```python
from build123d import *

# Parameters (mm, degrees)
CROQUIS1_W              = 20
CROQUIS1_H              = 60
SALIENTE_EXTRUIR1_DEPTH = 31
CORTAR_EXTRUIR1_REACH   = 72.434
CROQUIS2_W              = 21
CROQUIS2_H              = 50
CORTAR_EXTRUIR2_REACH   = 72.434
CROQUIS3_W              = 5
CROQUIS3_H              = 2
CORTAR_EXTRUIR3_REACH   = 72.434
CROQUIS4_W              = 7
CROQUIS4_H              = 2


with BuildPart() as part:
    # Croquis1 → Saliente-Extruir1 (new body)
    with BuildSketch(Plane.XY):
        with Locations((10, 30)):
            Rectangle(CROQUIS1_W, CROQUIS1_H)
    extrude(amount=SALIENTE_EXTRUIR1_DEPTH)

    # Croquis2 → Cortar-Extruir1 (cut, up to next)
    with BuildSketch(Plane(origin=(20, 0, 0), x_dir=(0, 0, -1), z_dir=(1, 0, 0)), mode=Mode.PRIVATE) as cortar_extruir1_sk1:
        with Locations((-20.5, 25)):
            Rectangle(CROQUIS2_W, CROQUIS2_H)
    cortar_extruir1_tool1 = extrude(cortar_extruir1_sk1.sketch, amount=-CORTAR_EXTRUIR1_REACH, mode=Mode.PRIVATE) & part.part
    add(cortar_extruir1_tool1.solids().sort_by_distance((20, 25, 20.5))[0], mode=Mode.SUBTRACT)

    # Croquis3 → Cortar-Extruir2 (cut, up to next)
    with BuildSketch(Plane(origin=(20, 0, 0), x_dir=(0, 0, -1), z_dir=(1, 0, 0)), mode=Mode.PRIVATE) as cortar_extruir2_sk1:
        with Locations((-28.5, 52.783625731)):
            Rectangle(CROQUIS3_W, CROQUIS3_H)
    cortar_extruir2_tool1 = extrude(cortar_extruir2_sk1.sketch, amount=-CORTAR_EXTRUIR2_REACH, mode=Mode.PRIVATE) & part.part
    add(cortar_extruir2_tool1.solids().sort_by_distance((20, 52.783626, 28.5))[0], mode=Mode.SUBTRACT)

    # Croquis4 → Cortar-Extruir3 (cut, up to next)
    with BuildSketch(Plane(origin=(20, 0, 0), x_dir=(0, 0, -1), z_dir=(1, 0, 0)), mode=Mode.PRIVATE) as cortar_extruir3_sk1:
        with Locations((-6.5, 4)):
            Rectangle(CROQUIS4_W, CROQUIS4_H)
    cortar_extruir3_tool1 = extrude(cortar_extruir3_sk1.sketch, amount=-CORTAR_EXTRUIR3_REACH, mode=Mode.PRIVATE) & part.part
    add(cortar_extruir3_tool1.solids().sort_by_distance((20, 4, 6.5))[0], mode=Mode.SUBTRACT)


solid = part.part
```
Model file for the job. Use its own axes, mm. A direction names the side the tool comes from. Give positions to 0.01 mm unless a question says otherwise; leave off trailing zeros. Write each loop counter-clockwise with the first axis right and the second up, starting at its lowest first coordinate (ties: lowest second). Pieces come first, ordered by that corner, then holes. Notation, with made-up numbers: (-22.5, 21.25) -> (-8.5, 21.25) arc R18 cw to (-8.5, 48.25) -> close; hole circle Ø8 at (10.25, -19.75). An arc over 180 degrees is marked (long way). Use CSV: the item, a comma, the result in double quotes. Start each with the question number.
1) Cut at D-D on z = 19. List the corners of the cut face in (x, y).
2) Cut at C-C on y = 53. List the corners of the cut face in (x, z), plus the area to 3 significant figures.
3) Cut at A-A on z = 6. List the corners of the cut face in (x, y), plus the area to 3 significant figures.
4) Tool access for faces 1 (the flat face through (10, 4, 3)), 2 (the flat face through (10, 57, 31)), 3 (the flat face through (10, 27, 10)): list every direction of +Z, -Z, +X, -X, +Y, -Y with a clear straight run to the whole face (end or side of a thin tool).
5) Drill centre lines: L1, parallel to Y at x = 14.25, z = 5; L2, parallel to Y at x = 11, z = 24.5; L3, parallel to Z at x = 8.5, y = 21. Where is each one in solid material? Low to high.
6) Two-plate mould, pull along Y, no slides. Class faces 4 (the flat face through (10, 60, 15)), 5 (the flat face through (10, 53, 26)), 6 (the flat face through (0, 36, 8)): released by +Y, released by -Y, zero draft, split by the parting line, or undercut.
7) Cut at B-B on x = 17. List the corners of the cut face in (y, z), plus the area to 3 significant figures.
8) Pin check, flat tips, straight feed: P1, Ø5.5, axis at x = 11.5, z = 28.5, coming from the -Y side; P2, Ø0.6, axis at x = 9.5, y = 52.5, coming from the +Z side; P3, Ø10, axis at y = 38, z = 19, coming from the +X side; P4, Ø1.5, axis at x = 7.5, y = 2, coming from the +Z side. Stop position of each tip, or through.
Final values:
1,outline,"(0, 50) -> (20, 50) -> (20, 60) -> (0, 60) -> close"
2,outline,"(0, 0) -> (20, 0) -> (20, 26) -> (0, 26) -> close"
2,area,"520 mm2"
3,outline,"(0, 0) -> (20, 0) -> (20, 3) -> (0, 3) -> close; (0, 5) -> (20, 5) -> (20, 60) -> (0, 60) -> close"
3,area,"1,160 mm2"
4,face 1,"+Z, +X, -X"
4,face 2,"+Z, +X, -X, +Y, -Y"
4,face 3,"+Z, +X, -X, -Y"
5,L1,"y = 0 to 3, 5 to 60"
5,L2,"y = 50 to 60"
5,L3,"z = 0 to 10"
6,face 4,"released by +Y"
6,face 5,"undercut"
6,face 6,"zero draft"
7,outline,"(0, 0) -> (60, 0) -> (60, 31) -> (53.78, 31) -> (53.78, 26) -> (51.78, 26) -> (51.78, 31) -> (50, 31) -> (50, 10) -> (5, 10) -> (5, 3) -> (3, 3) -> (3, 10) -> (0, 10) -> close"
7,area,"786 mm2"
8,P1,"stops at y = 50"
8,P2,"stops at z = 26"
8,P3,"passes through"
8,P4,"stops at z = 10"
